Check sheet for the modelled part. Datum: model origin and axes. Units: mm. A direction names the side the tool comes from. Round coordinates to 2 decimals unless told otherwise and drop trailing zeros. Loops run counter-clockwise (first coordinate to the right, second up) from the corner with the lowest first, then second, coordinate; pieces in that order, holes last. Notation, with made-up numbers: (76, 11) -> (125, 11) arc R22 cw to (125, 21) -> close; hole circle Ø2 at (43, -6.75). An arc over 180 degrees is marked (long way). One line per question, with ' | ' between items.
Solid Edge part; units mm, degrees
sketch "Sketch1" plane through (0, 0, 0) normal (0, 0, 1) x (1, 0, 0)
  line L0 (2.5, 0) -> (2.5, 20)
  line L1 (0, 20) -> (2.5, 20)
  line L2 (0, 0) -> (0, 20)
  line L3 (0, 0) -> (0, -2.75)
  line L4 (0, -2.75) -> (4.75, -2.75)
  line L5 (4.75, -2.75) -> (4.75, 0)
  line L6 (4.75, 0) -> (2.5, 0)
revolve "RevolvedProtrusion1" add sketch "Sketch1" angle 360 about axis through (0, 0, 0) along (0, 1, 0)
sketch "Sketch2" plane through (0, 0, 0) normal (1, 0, 0) x (0, 1, 0)
  line L0 (-2.75, 2.2215) -> (-1.19, 2.2215)
  line L1 (0.0926, 0) -> (-1.19, 2.2215)
  line L2 (-2.75, 0) -> (0.0926, 0)
  line L3 (-2.75, 0) -> (-2.75, 2.2215)
revolve "RevolvedCutout1" cut sketch "Sketch2" angle 360 about axis through (0, -4.5, 0) along (0, 1, 0)
sketch "Sketch3" plane through (0, -2.75, 0) normal (0, -1, 0) x (0, 0, 1)
  circle A0 centre (0, 0) radius 2.2215
  line L0 (-1.5, -0.866) -> (0, -1.7321)
  line L1 (0, -1.7321) -> (1.5, -0.866)
  line L2 (1.5, -0.866) -> (1.5, 0.866)
  line L3 (1.5, 0.866) -> (0, 1.7321)
  line L4 (0, 1.7321) -> (-1.5, 0.866)
  line L5 (-1.5, 0.866) -> (-1.5, -0.866)
extrude "Protrusion1" add sketch "Sketch3" against normal up to next
sketch "Sketch4" plane through (0, 0, 0) normal (0, 0, 1) x (1, 0, 0)
  line L0 (-1.7321, -2.75) -> (0, -2.75)
  line L1 (0, -2.75) -> (0, -2.2859)
  line L2 (0, -2.2859) -> (-1.7321, -2.75)
revolve "RevolvedCutout2" cut sketch "Sketch4" angle 360 about axis through (0, -4.5, 0) along (0, 1, 0)
fillet "Round1" radius 0.2 1 edges at (0, 0, -2.5)
chamfer "倒斜角_2" distance 0.3333 angle 45 1 edges at (0, 20, -2.5)
cosmetic_thread "螺纹_3" thread depth 18.4
sketch "Sketch5" plane through (0, 0, 0) normal (0, 0, 1) x (1, 0, 0)
  arc A0 (-2.2953, -2.75) -> (-4.75, 0) centre (-1.9822, 0) cw
revolve "RevolvedCutout3" cut sketch "Sketch5" angle 360 about axis through (0, 0, 0) along (0, -1, 0) material side at (-4.0844, -1.8764, 0)
properties part number "N2611-1122" material "铝 1060"
(1) Go/stop test with flat-tipped pins: pin 1 (1 mm diameter, centred on x = 2.5, z = 3.5, fed in from +Y); pin 2 (0.9 mm diameter, centred on x = 0.5, y = -2, fed in from -Z); pin 3 (1.4 mm diameter, centred on x = 0, y = -2, fed in from +Z). Record where each tip stops, or that it passes through.
Answer:
pin 1: stops at y = 0 | pin 2: stops at z = -4.25 | pin 3: stops at z = 4.43
(2) Mould release check, pull along Z, two halves, no side actions. Record for faces 3 (the face through (0.11, 0.03, -0.02)), 4 (the face through (2.04, 0, 2.04)), 5 (the face through (-0.54, 10.07, 2.44)): +Z half, -Z half, draft (parallel to the pull), parting line (faces both ways), or undercut.
Answer:
face 3: undercut | face 4: draft | face 5: parting line
(3) Set-up check for faces 1 (the face through (0, 20, 0)), 2 (the face through (0, -2, 1.5)): record each of +Z, -Z, +X, -X, +Y, -Y from which the full face is reachable in a straight line by a thin tool's end or side.
Answer:
face 1: +Z, -Z, +X, -X, +Y | face 2: -Y
(4) Scan lines: probe 1 along X at (y, z) = (5.75, 2); probe 2 along Z at (x, y) = (1, 14.25). Record each from-to range of solid material in increasing order.
Answer:
probe 1: x = -1.5 to 1.5 | probe 2: z = -2.29 to 2.29
(5) Sectioned sample at A-A, the plane y = 6. Record the cut outline in (x, z), and give its area (3 significant figures).
Answer:
outline: circle Ø5 at (0, 0) | area: 19.6 mm2
